from build123d import *

# Parameters (mm, degrees)
SKETCH2_R           = 2.1
BOSS_EXTRUDE1_DEPTH = 1.5748
SKETCH3_W           = 12
SKETCH3_H           = 25.4
SKETCH3_W_2         = 10
SKETCH3_H_2         = 12
BOSS_EXTRUDE2_DEPTH = 5
SKETCH5_W           = 15
SKETCH5_H           = 15
BOSS_EXTRUDE3_DEPTH = 13.4252


with BuildPart() as part:
    # Sketch2 → Boss-Extrude1 (new body)
    with BuildSketch(Plane(origin=(0, 0, 0), x_dir=(1, 0, 0), z_dir=(0, 1, 0))):
        with BuildLine():
            Line((5, 0), (135, 0))
            ThreePointArc((135, 0), (138.535533906, 1.464466094), (140, 5))
            Line((140, 5), (140, 55))
            ThreePointArc((140, 55), (138.535533906, 58.535533906), (135, 60))
            Line((135, 60), (5, 60))
            ThreePointArc((5, 60), (1.464466094, 58.535533906), (0, 55))
            Line((0, 55), (0, 5))
            ThreePointArc((0, 5), (1.464466094, 1.464466094), (5, 0))
        make_face()
        with Locations(Location((5, 55, 0), (0, 0, 270))):
            Circle(SKETCH2_R, mode=Mode.SUBTRACT)
        with Locations(Location((5, 5, 0), (0, 0, 270))):
            Circle(SKETCH2_R, mode=Mode.SUBTRACT)
        with Locations(Location((135, 5, 0), (0, 0, 270))):
            Circle(SKETCH2_R, mode=Mode.SUBTRACT)
        with Locations(Location((135, 55, 0), (0, 0, 270))):
            Circle(SKETCH2_R, mode=Mode.SUBTRACT)
        with Locations(Location((78.249999964, 55, 0), (0, 0, 270))):
            Circle(SKETCH2_R, mode=Mode.SUBTRACT)
        with Locations(Location((78.249999964, 5, 0), (0, 0, 270))):
            Circle(SKETCH2_R, mode=Mode.SUBTRACT)
    extrude(amount=BOSS_EXTRUDE1_DEPTH)

    # Sketch3 → Boss-Extrude2 (add)
    with BuildSketch(Plane(origin=(0, 1.5748, 0), x_dir=(1, 0, 0), z_dir=(0, 1, 0))):
        with Locations((136, 30)):
            Rectangle(SKETCH3_W, SKETCH3_H)
        with Locations((40, 53)):
            Rectangle(SKETCH3_W_2, SKETCH3_H_2)
        with Locations((27, 53)):
            Rectangle(SKETCH3_W_2, SKETCH3_H_2)
    extrude(amount=BOSS_EXTRUDE2_DEPTH)

    # Sketch5 → Boss-Extrude3 (add)
    with BuildSketch(Plane(origin=(0, 1.5748, 0), x_dir=(1, 0, 0), z_dir=(0, 1, 0))):
        with Locations((84.749999964, 40.5)):
            Rectangle(SKETCH5_W, SKETCH5_H)
    extrude(amount=BOSS_EXTRUDE3_DEPTH)


solid = part.part
Input: part model. Units: mm. Frame: model coordinates. A direction names the side the tool comes from. Coordinates: 2 decimals unless noted, no trailing zeros. Order: outer loops, then holes, each group sorted by start corner. A loop starts at its lowest first (then second) coordinate and runs counter-clockwise, first axis right, second up. Notation, with made-up numbers: M 0,-38.5 L 37,-38.5 A13 cw 37,-20.5 Z; hole C 57.25,71.25 d1. An arc over 180 degrees is marked long. Answer in a Markdown table with one row per item.
(1) Section query D-D, the plane x = 111. Output: boundary loops of the cut face in (y, z).
Numbers:
| item | result |
|---|---|
| outline | M 0,-60 L 1.57,-60 L 1.57,0 L 0,0 Z |
(2) Section query A-A, the plane z = -23.5. Output: boundary loops of the cut face in (x, y), plus the area to 3 significant figures.
Numbers:
| item | result |
|---|---|
| outline | M 0,0 L 140,0 L 140,1.57 L 142,1.57 L 142,6.57 L 130,6.57 L 130,1.57 L 0,1.57 Z |
| area | 280 mm^2 |
(3) Section query B-B, the plane x = 38. Output: boundary loops of the cut face in (y, z), plus the area to 3 significant figures.
Numbers:
| item | result |
|---|---|
| outline | M 0,-60 L 1.57,-60 L 1.57,-59 L 6.57,-59 L 6.57,-47 L 1.57,-47 L 1.57,0 L 0,0 Z |
| area | 154 mm^2 |
(4) Material intervals for line 1 (X direction, y = 0.95, z = -5); line 2 (Z direction, x = 135, y = 0.7); line 3 (X direction, y = 3.5, z = -56), sorted ascending. Write a range as [from, to].
Numbers:
| item | result |
|---|---|
| line 1 | x = [0, 2.9], [7.1, 76.15], [80.35, 132.9], [137.1, 140] |
| line 2 | z = [-60, -57.1], [-52.9, -7.1], [-2.9, 0] |
| line 3 | x = [22, 32], [35, 45] |
(5) Draft query along X for faces 6 (the flat face through (40, 4, -47)), 7 (the flat face through (92.25, 8, -40)), 8 (the flat face through (142, 4, -30)). Return one class per face: pulls with the +X half, pulls with the -X half, needs draft (parallel to the pull), parting line crosses it, or undercut.
Numbers:
| item | result |
|---|---|
| face 6 | needs draft |
| face 7 | undercut |
| face 8 | pulls with the +X half |
(6) Section query C-C, the plane y = 11. Output: boundary loops of the cut face in (x, z), plus the area to 3 significant figures.
Numbers:
| item | result |
|---|---|
| outline | M 77.25,-48 L 92.25,-48 L 92.25,-33 L 77.25,-33 Z |
| area | 225 mm^2 |
(7) Access query for faces 1 (the flat face through (85, 8, -48)), 2 (the cylindrical face through (139, 1, -58)), 3 (the flat face through (136, 6.575, -30)), 4 (the flat face through (32, 4, -53)), 5 (the flat face through (27, 4, -59)). Directions: +Z, -Z, +X, -X, +Y, -Y. A direction counts if a zero-diameter tool reaches every point of the face in a straight line with its end or side. Return the directions, or none.
Numbers:
| item | result |
|---|---|
| face 1 | -Z, +X, +Y |
| face 2 | -Z, +X, +Y, -Y |
| face 3 | +Z, -Z, +X, +Y |
| face 4 | +Z, -Z, +Y |
| face 5 | -Z, +X, -X, +Y |
(8) Contact query for flat-ended pins moving along their axis: pin 1 Ø1.7 at (y, z) = (0.5, -27) entering from +X; pin 2 Ø1 at (x, z) = (100.5, -25.5) entering from +Y; pin 3 Ø1.5 at (y, z) = (3.5, -42) entering from -X; pin 4 Ø3.5 at (x, z) = (5, -5) entering from +Y. Output: stop coordinate, or through.
Numbers:
| item | result |
|---|---|
| pin 1 | stops at x = 140 |
| pin 2 | stops at y = 1.57 |
| pin 3 | stops at x = 77.25 |
| pin 4 | passes through |
